```python
from build123d import *

# Parameters (mm, degrees)
BOSS_EXTRUDE1_DEPTH      = 141
BOSS_EXTRUDE1_DEPTH_BACK = 141
SKETCH1_W                = 22
SKETCH1_H                = 100
CAVITY1_START            = -2
CAVITY1_OUTLINE_W        = 282
CAVITY1_OUTLINE_H        = 40
CAVITY1_DEPTH            = 2


# Read off the part's stored shape, not the designer's step: Cavity1
with BuildPart() as part:
    # Sketch1 → Boss-Extrude1 (new, two sides: drawn at the far end of the back side and taken through both)
    with BuildSketch(Plane(origin=(0, 0, 0), x_dir=(0, 0, -1), z_dir=(1, 0, 0)).offset(-BOSS_EXTRUDE1_DEPTH_BACK)):
        with Locations((1, -190)):
            Rectangle(SKETCH1_W, SKETCH1_H)
    extrude(amount=BOSS_EXTRUDE1_DEPTH + BOSS_EXTRUDE1_DEPTH_BACK)

    # Cavity1 outline → Cavity1 (cut)
    with BuildSketch(Plane.XY.offset(CAVITY1_START)):
        with Locations((0, -160)):
            Rectangle(CAVITY1_OUTLINE_W, CAVITY1_OUTLINE_H)
    cavity1 = extrude(amount=CAVITY1_DEPTH, mode=Mode.SUBTRACT)

    # Mirror1: Cavity1 across plane
    add(cavity1.mirror(Plane.ZX.offset(-190)), mode=Mode.SUBTRACT)


solid = part.part
```
The listing builds one solid part. Answer for the finished solid, in the listing's coordinates (mm). A direction names the side the tool comes from. Coordinates: 2 decimals unless noted, no trailing zeros. Loops run counter-clockwise (first coordinate to the right, second up) from the corner with the lowest first, then second, coordinate; pieces in that order, holes last. Notation, with made-up numbers: (57, 84.25) -> (87, 84.25) arc R10 cw to (87, 100.25) -> close; hole circle Ø7 at (-18.5, 58). An arc over 180 degrees is marked (long way). Return JSON: item names as keys, results as strings. Group by question number.
(1) A cutting plane is placed at A-A on y = -212. Write down the section's boundary in (x, z), and give its area (3 significant figures).
(2) Determine the mould class of faces 4 (the flat face through (-2, -220, 0)), 5 (the flat face through (-2, -140, 5)), 6 (the flat face through (-2, -191, -12)) for opening direction Z: released by +Z, released by -Z, zero draft, split by the parting line, or undercut.
(3) A cutting plane is placed at B-B on x = -98.5. Write down the section's boundary in (y, z), and give its area (3 significant figures).
(4) Given pin 1 Ø1.6 at (x, z) = (20, -1) entering from -Y, flat-ended and moving along its own axis, determine where the tip first touches the part or whether it passes through.
(5) Find the intervals of material crossed by probe 1 along Z at (x, y) = (53.5, -221); probe 2 along Y at (x, z) = (57.5, -1.75), in increasing order. Write a range as from..to.
(6) Which of the six approach directions +Z, -Z, +X, -X, +Y, -Y give full straight-line access (tool end or side, diameter ignored) to faces 1 (the flat face through (-2, -160, -2)), 2 (the flat face through (-2, -140, -7)), 3 (the flat face through (-2, -220, -2))?
The answers:
{
 "1": {"outline": "(-141, -12) -> (141, -12) -> (141, -2) -> (-141, -2) -> close; (-141, 0) -> (141, 0) -> (141, 10) -> (-141, 10) -> close", "area": "5,640 mm^2"},
 "2": {"face 4": "undercut", "face 5": "zero draft", "face 6": "released by -Z"},
 "3": {"outline": "(-240, -12) -> (-140, -12) -> (-140, -2) -> (-180, -2) -> (-180, 0) -> (-140, 0) -> (-140, 10) -> (-240, 10) -> (-240, 0) -> (-200, 0) -> (-200, -2) -> (-240, -2) -> close", "area": "2,040 mm^2"},
 "4": {"pin 1": "stops at y = -200"},
 "5": {"probe 1": "z = -12..-2, 0..10", "probe 2": "y = -200..-180"},
 "6": {"face 1": "+X, -X, +Y", "face 2": "+Z, -Z, +X, -X, +Y", "face 3": "+X, -X, -Y"}
}
